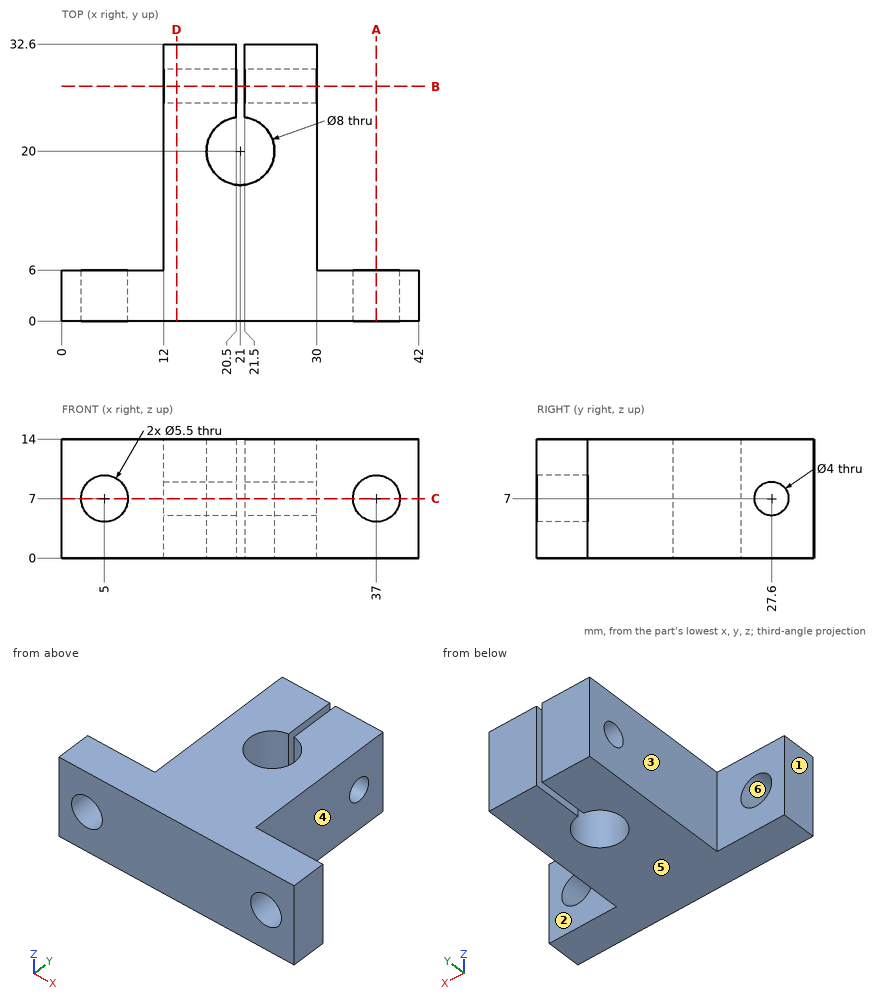
Geometry check sheet. Reference: drawing and pictorial views, mm from the part's lowest x, y, z. A direction names the side the tool comes from. Give positions to 0.01 mm unless a question says otherwise; leave off trailing zeros. Order: outer loops, then holes, each group sorted by start corner. A loop starts at its lowest first (then second) coordinate and runs counter-clockwise, first axis right, second up. Notation, with made-up numbers: M 88.25,74 L 138.25,74 A18 ccw 138.25,97 Z; hole C 72.5,-1 d4. An arc over 180 degrees is marked long. Return JSON: item names as keys, results as strings. Group by question number.
1) Go/stop test with flat-tipped pins: pin 1 Ø7 at (y, z) = (27, 4.5) entering from -X; pin 2 Ø6 at (x, z) = (35.5, 8) entering from +Y; pin 3 Ø7 at (y, z) = (28.5, 10) entering from +X. Record where each tip stops, or that it passes through.
2) Section check B-B on y = 27.6. Record the cut outline in (x, z).
3) Section check C-C on z = 7. Record the cut outline in (x, y), and give its area (3 significant figures).
4) Section check A-A on x = 37. Record the cut outline in (y, z), and give its area (3 significant figures).
5) Section check D-D on x = 13.5. Record the cut outline in (y, z).
6) Access from +Z, -Z, +X, -X, +Y, -Y to the whole of each face (thin tool, end or side, straight path). Record for the marked faces 1, 2 and 3.
7) Mould release check, pull along X, two halves, no side actions. Record for the marked faces 4, 5 and 6: pulls with the +X half, pulls with the -X half, needs draft (parallel to the pull), parting line crosses it, or undercut.
8) Scan lines: line 1 (Y direction, x = 27, z = 7); line 2 (X direction, y = 3.7, z = 7); line 3 (X direction, y = 24.5, z = 12.25). Record each from-to range of solid material in increasing order.
Answer block:
{
 "1": {"pin 1": "stops at x = 12", "pin 2": "stops at y = 6", "pin 3": "stops at x = 30"},
 "2": {"outline": "M 12,0 L 20.5,0 L 20.5,5 L 12,5 Z; M 12,9 L 20.5,9 L 20.5,14 L 12,14 Z; M 21.5,0 L 30,0 L 30,5 L 21.5,5 Z; M 21.5,9 L 30,9 L 30,14 L 21.5,14 Z"},
 "3": {"outline": "M 0,0 L 2.25,0 L 2.25,6 L 0,6 Z; M 7.75,0 L 34.25,0 L 34.25,6 L 30,6 L 30,25.6 L 21.5,25.6 L 21.5,23.97 A4 cw long 20.5,23.97 L 20.5,25.6 L 12,25.6 L 12,6 L 7.75,6 Z; M 12,29.6 L 20.5,29.6 L 20.5,32.6 L 12,32.6 Z; M 21.5,29.6 L 30,29.6 L 30,32.6 L 21.5,32.6 Z; M 39.75,0 L 42,0 L 42,6 L 39.75,6 Z", "area": "538 mm^2"},
 "4": {"outline": "M 0,0 L 6,0 L 6,4.25 L 0,4.25 Z; M 0,9.75 L 6,9.75 L 6,14 L 0,14 Z", "area": "51.0 mm^2"},
 "5": {"outline": "M 0,0 L 32.6,0 L 32.6,14 L 0,14 Z; hole C 27.6,7 d4"},
 "6": {"face 1": "+Z, -Z, -X, +Y, -Y", "face 2": "+Z, -Z, +X, +Y", "face 3": "+Z, -Z, -X, +Y"},
 "7": {"face 4": "pulls with the +X half", "face 5": "needs draft", "face 6": "undercut"},
 "8": {"line 1": "y = 0 to 25.6, 29.6 to 32.6", "line 2": "x = 0 to 2.25, 7.75 to 34.25, 39.75 to 42", "line 3": "x = 12 to 20.5, 21.5 to 30"}
}
